```python
from build123d import *

# Parameters (mm, degrees)
F1_DEPTH = 25
F2_W     = 13.627150096
F2_H     = 15.5199997797
F3_DEPTH = 25
F4_R     = 3.852849114
F5_DEPTH = 25


with BuildPart() as f1:
    # F0 (on Front) → F1 (new body)
    with BuildSketch(Plane.XZ):
        Polygon((-27.6273339987, 13.7823959813), (-40.0947295129, 30.5988863111), (-49.6627315879, 13.7823959813), align=None)
    extrude(amount=-F1_DEPTH)

    # F2 (on face) → F3 (cut)
    with BuildSketch(Plane(origin=(-11.2344276136, 0, -8.3289705336), x_dir=(0, 1, 0), z_dir=(0.8033118285, 0, 0.5955586505))):
        with Locations((12.2393383645, 40.6992104239)):
            Rectangle(F2_W, F2_H)
    extrude(amount=-F3_DEPTH, mode=Mode.SUBTRACT)


with BuildPart() as f5:
    # F4 (on Right) → F5 (new body)
    with BuildSketch(Plane.YZ):
        with Locations((-33.5409045219, 28.1745772809)):
            Circle(F4_R)
    extrude(amount=-F5_DEPTH)


solid = f1.part
```
Geometry check sheet. Reference: the model listing, model coordinates, mm. A direction names the side the tool comes from. Round coordinates to 2 decimals unless told otherwise and drop trailing zeros. Order: outer loops, then holes, each group sorted by start corner. A loop starts at its lowest first (then second) coordinate and runs counter-clockwise, first axis right, second up. Notation, with made-up numbers: (85.5, 21.5) - (95.5, 21.5) arc R26 cw to (95.5, 48.5) - close; hole circle Ø10 at (43, 71.25). An arc over 180 degrees is marked (long way). Use a Markdown table: item, result. Add a question column.
1) Gauge pin test, flat ends, axial feed: P1, Ø3, axis at y = 13.5, z = 20, coming from the +X side; P2, Ø6, axis at y = 21.5, z = 26.5, coming from the +X side; P3, Ø5, axis at y = 21.5, z = 24.5, coming from the +X side; P4, Ø1, axis at x = -41.5, y = 3.5, coming from the +Z side. Record the tip position at first contact, or that the pin passes through.
2) Section check C-C (y = 22.75). Record the cut outline in (x, z), then the cut area to 3 significant figures.
3) Thickness scan on line 1 along Y through (x, z) = (-33, 19); line 2 along X through (y, z) = (20, 26.5); line 3 along Z through (x, y) = (-47.5, 3.25). Record the ranges inside material, lowest first.
4) Mould release check, pull along Y, two halves, no side actions. Record for faces 1 (the flat face through (-41, 19.053, 20)), 2 (the flat face through (-39, 25, 19)), 3 (the flat face through (-29.62, 12.32, 16.47)): released by +Y, released by -Y, zero draft, split by the parting line, or undercut.
5) Section check D-D (z = 17). Record the cut outline in (x, y).
6) Section check A-A (z = 28.5). Record the cut outline in (x, y).
7) Section check B-B (x = -42.5). Record the cut outline in (y, z), then the cut area to 3 significant figures.
8) Set-up check for faces 4 (the flat face through (-41, 5.426, 20)), 5 (the flat face through (-39, 0, 19)): record each of +Z, -Z, +X, -X, +Y, -Y from which the full face is reachable in a straight line by a thin tool's end or side.
Established:
| question | item | result |
|---|---|---|
| 1 | P1 | through |
| 1 | P2 | x = -34.83 |
| 1 | P3 | x = -33.72 |
| 1 | P4 | z = 29.01 |
| 2 | outline | (-49.66, 13.78) - (-27.63, 13.78) - (-40.09, 30.6) - close |
| 2 | area | 185 mm2 |
| 3 | line 1 | 0 to 5.43, 19.05 to 25 |
| 3 | line 2 | -42.43 to -37.06 |
| 3 | line 3 | 13.78 to 17.58 |
| 4 | face 1 | undercut |
| 4 | face 2 | released by +Y |
| 4 | face 3 | zero draft |
| 5 | outline | (-47.83, 0) - (-30.01, 0) - (-30.01, 25) - (-47.83, 25) - (-47.83, 19.05) - (-32.38, 19.05) - (-32.38, 5.43) - (-47.83, 5.43) - close |
| 6 | outline | (-41.29, 0) - (-38.54, 0) - (-38.54, 5.43) - (-41.29, 5.43) - close; (-41.29, 19.05) - (-38.54, 19.05) - (-38.54, 25) - (-41.29, 25) - close |
| 7 | outline | (0, 13.78) - (5.43, 13.78) - (5.43, 26.37) - (0, 26.37) - close; (19.05, 13.78) - (25, 13.78) - (25, 26.37) - (19.05, 26.37) - close |
| 7 | area | 143 mm2 |
| 8 | face 4 | +Z, -X |
| 8 | face 5 | +Z, -Z, +X, -X, -Y |
